```python
from build123d import *

# Parameters (mm, degrees)
CROQUIS1_W                 = 117
CROQUIS1_H                 = 200
SALIENTE_EXTRUIR1_DEPTH    = 5
CROQUIS2_W                 = 127
CROQUIS2_H                 = 210
CROQUIS2_W_2               = 117
CROQUIS2_H_2               = 200
SALIENTE_EXTRUIR2_DEPTH    = 150
CROQUIS3_W                 = 100
CROQUIS3_H                 = 210
SALIENTE_EXTRUIR3_DEPTH    = 40
SALIENTE_EXTRUIR4_DEPTH    = 167
REDONDEO1_R                = 15
CORTAR_EXTRUIR1_DEPTH      = 207.790352773
CORTAR_EXTRUIR1_DEPTH_BACK = 30
CROQUIS5_W                 = 30
CROQUIS5_H                 = 210
CROQUIS6_W                 = 12.5
CROQUIS6_H                 = 8.471901852
CROQUIS6_R                 = 2.5
SALIENTE_EXTRUIR6_DEPTH    = 2


with BuildPart() as part:
    # Croquis1 → Saliente-Extruir1 (new body)
    with BuildSketch(Plane.XY):
        Rectangle(CROQUIS1_W, CROQUIS1_H)
    extrude(amount=SALIENTE_EXTRUIR1_DEPTH)

    # Croquis2 → Saliente-Extruir2 (add)
    with BuildSketch(Plane.XY.offset(5)):
        Rectangle(CROQUIS2_W, CROQUIS2_H)
        Rectangle(CROQUIS2_W_2, CROQUIS2_H_2, mode=Mode.SUBTRACT)
    extrude(amount=-SALIENTE_EXTRUIR2_DEPTH)

    # Croquis3 → Saliente-Extruir3 (add)
    with BuildSketch(Plane.ZY.offset(63.5)):
        with Locations((-45, 0)):
            Rectangle(CROQUIS3_W, CROQUIS3_H)
    extrude(amount=SALIENTE_EXTRUIR3_DEPTH)

    # Croquis4 → Saliente-Extruir4 (add)
    with BuildSketch(Plane.ZY.offset(103.5)):
        with BuildLine():
            Line((5, 105), (5, -105))
            ThreePointArc((5, -105), (25, 0), (5, 105))
        make_face()
    extrude(amount=-SALIENTE_EXTRUIR4_DEPTH)

    # Redondeo1
    redondeo1_edges = [part.edges().sort_by_distance(p)[0] for p in [
        (63.5, 105, -70),
        (63.5, -105, -70),
        (-63.5, -105, -120),
        (-63.5, 105, -120),
        (-20, 105, 5),
        (-20, -105, 5),
        (-63.5, 0, -95),
        (-83.5, 105, -95),
        (-83.5, -105, -95),
        (-103.5, 105, -45),
        (-103.5, 0, -95),
        (-103.5, -105, -45),
        (-103.5, 0, 25),
        (63.5, 0, 25),
    ]]
    fillet(redondeo1_edges, radius=REDONDEO1_R)

    # Croquis5 → Cortar-Extruir1 (cut, two sides: drawn at the far end of the back side and taken through both)
    with BuildSketch(Plane.XY.offset(-CORTAR_EXTRUIR1_DEPTH_BACK)):
        with Locations((-73.5, 0)):
            Rectangle(CROQUIS5_W, CROQUIS5_H)
    extrude(amount=CORTAR_EXTRUIR1_DEPTH + CORTAR_EXTRUIR1_DEPTH_BACK, mode=Mode.SUBTRACT)

    # Croquis6 → Saliente-Extruir6 (add)
    # profile 1 of 2: a face of its own
    with BuildSketch(Plane.ZY.offset(58.5)):
        with Locations((-6.25, -40.416867006)):
            Rectangle(CROQUIS6_W, CROQUIS6_H)
        with Locations((-7.403741824, -40.5)):
            Circle(CROQUIS6_R, mode=Mode.SUBTRACT)
    # profile 2 of 2: a face of its own
    with BuildSketch(Plane.ZY.offset(58.5)):
        with Locations((-6.25, -89.583132994)):
            Rectangle(CROQUIS6_W, CROQUIS6_H)
        with Locations((-7.403741824, -89.5)):
            Circle(CROQUIS6_R, mode=Mode.SUBTRACT)
    extrude(amount=-SALIENTE_EXTRUIR6_DEPTH)


solid = part.part
```
Model file for the job. Use its own axes, mm. A direction names the side the tool comes from. Round coordinates to 2 decimals unless told otherwise and drop trailing zeros. Write each loop counter-clockwise with the first axis right and the second up, starting at its lowest first coordinate (ties: lowest second). Pieces come first, ordered by that corner, then holes. Notation, with made-up numbers: (74.5, 32) - (115.5, 32) arc R14 cw to (115.5, 44) - close; hole circle Ø8 at (-26.75, 38.25). An arc over 180 degrees is marked (long way). Use CSV: the item, a comma, the result in double quotes. Start each with the question number.
Item 1: Drill centre lines: L1, parallel to X at y = -91, z = -11; L2, parallel to X at y = 39, z = -67; L3, parallel to Y at x = 39, z = -43. Where is each one in solid material? Low to high. Write a range as [from, to].
Item 2: Tool access for faces 5 (the face through (-58.5, 0, 8)), 6 (the face through (-56.5, -90.5, -4.9)), 7 (the face through (-63.5, -1, -127)): list every direction of +Z, -Z, +X, -X, +Y, -Y with a clear straight run to the whole face (end or side of a thin tool).
Item 3: Band-saw the part on C-C (x = -6). Write the cut outline in (y, z) (3 decimals), and give its area (3 significant figures).
Item 4: Band-saw the part on B-B (z = -129). Write the cut outline in (x, y).
Item 5: Pin check, flat tips, straight feed: P1, Ø3, axis at x = -84.5, y = -2.5, coming from the -Z side; P2, Ø17.5, axis at y = -34.5, z = -123, coming from the -X side; P3, Ø5, axis at x = -25.5, y = -61.5, coming from the -Z side; P4, Ø10, axis at x = -82, z = -10.5, coming from the -Y side. Stop position of each tip, or through.
Item 6: Two-plate mould, pull along X, no slides. Class faces 1 (the face through (-98.99, 100.72, -42.18)), 2 (the face through (58.5, -1, -71)), 3 (the face through (-4, 105, -76)), 4 (the face through (63.5, 1, -69)): released by +X, released by -X, zero draft, split by the parting line, or undercut.
Item 7: Band-saw the part on A-A (z = -20.5). Write the cut outline in (x, y), and give its area (3 significant figures).
Checked values:
1,L1,"x = [-103.47, -88.5], [-58.5, -56.5], [58.5, 63.47]"
1,L2,"x = [-103.5, -58.5], [58.5, 63.5]"
1,L3,"y = [-105, -100], [100, 105]"
2,face 5,"+Z, +Y, -Y"
2,face 6,"-Z"
2,face 7,"-Z, -X, +Y, -Y"
3,outline,"(-105, -145) - (-100, -145) - (-100, 0) - (100, 0) - (100, -145) - (105, -145) - (105, -5.404) arc R15 ccw to (94.988, 8.742) arc R285.625 ccw to (-94.988, 8.742) arc R15 ccw to (-105, -5.404) - close"
3,area,"5,280 mm²"
4,outline,"(-63.5, -90) arc R15 ccw to (-48.5, -105) - (48.5, -105) arc R15 ccw to (63.5, -90) - (63.5, 90) arc R15 ccw to (48.5, 105) - (-48.5, 105) arc R15 ccw to (-63.5, 90) - close; hole (-58.5, -100) - (58.5, -100) - (58.5, 100) - (-58.5, 100) - close"
5,P1,"stops at z = -95"
5,P2,"stops at x = -63.5"
5,P3,"stops at z = 0"
5,P4,"passes through"
6,face 1,"released by -X"
6,face 2,"undercut"
6,face 3,"zero draft"
6,face 4,"released by +X"
7,outline,"(-103.5, -90) arc R15 ccw to (-88.5, -105) - (-88.5, 105) arc R15 ccw to (-103.5, 90) - close; (-58.5, -105) - (48.5, -105) arc R15 ccw to (63.5, -90) - (63.5, 90) arc R15 ccw to (48.5, 105) - (-58.5, 105) - (-58.5, 100) - (58.5, 100) - (58.5, -100) - (-58.5, -100) - close"
7,area,"5,180 mm²"
